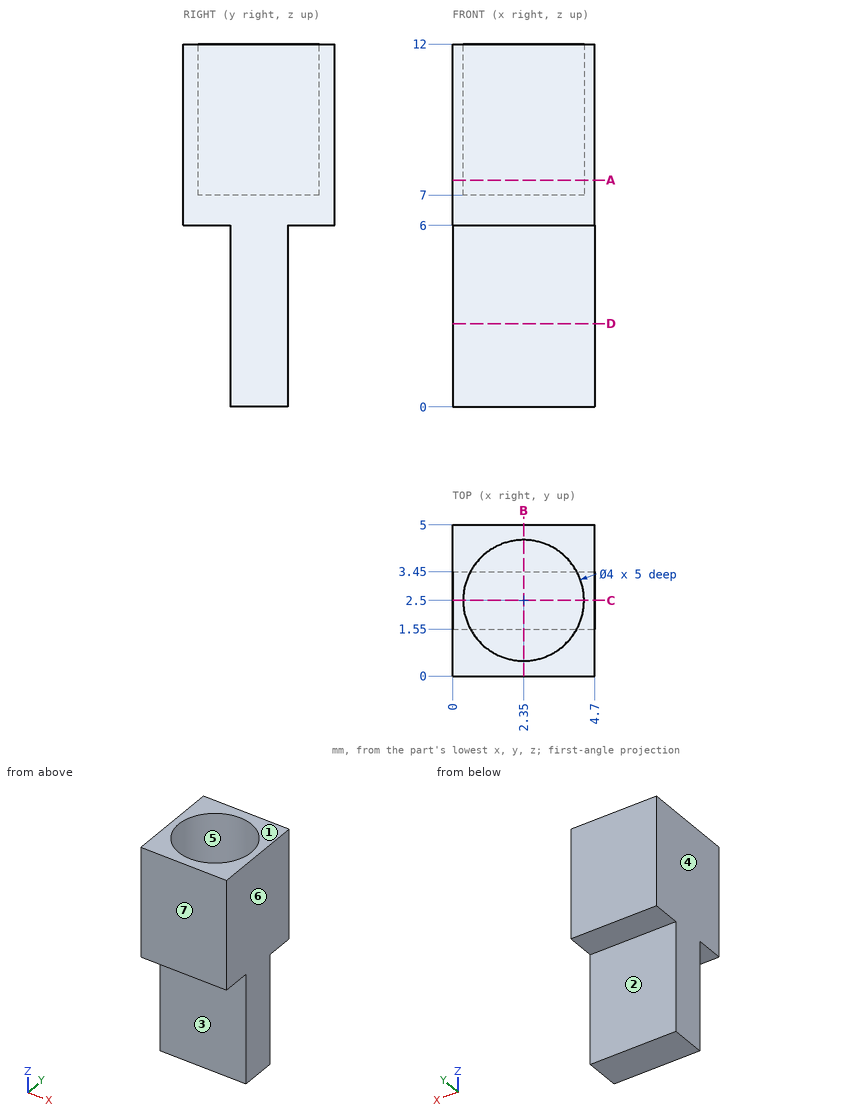
Here's the drawing with two shaded views (mm, measured from the low corner). I have some questions. A direction names the side the tool comes from. Give positions to 0.01 mm unless a question says otherwise; leave off trailing zeros. Order: outer loops, then holes, each group sorted by start corner. A loop starts at its lowest first (then second) coordinate and runs counter-clockwise, first axis right, second up. Notation, with made-up numbers: (-14.75, 83.25) -> (7.25, 83.25) arc R24 cw to (7.25, 98.25) -> close; hole circle Ø8 at (16.25, -6). An arc over 180 degrees is marked (long way). One line per item, written item: value. Start each with the question number.
1. Imagine slicing it at D-D, the plane z = 2.75. List the corners of the cut face in (x, y) for me.
2. Imagine slicing it at A-A, the plane z = 7.5. List the corners of the cut face in (x, y) for me.
3. I need wall thicknesses on probe 1 along Y at (x, z) = (2.35, 11); probe 2 along Z at (x, y) = (2.8, 0.7); probe 3 along Y at (x, z) = (0.8, 3.5). Which ranges of each line are inside material? Lowest first, please. Write a range as from..to.
4. For the marked faces 1, 2 and 3, which set-ups out of +Z, -Z, +X, -X, +Y, -Y let a thin tool reach every point of the face, with its end or its side?
5. Will these pins go through, and if not, where does the flat tip stop? pin 1 Ø1.5 at (x, y) = (3.5, 4.5) entering from -Z; pin 2 Ø2 at (x, z) = (3.5, 2.5) entering from +Y.
6. We'd pull the mould along X, two halves only. Please class the marked faces 4, 5, 6 and 7: released by +X, released by -X, zero draft, split by the parting line, or undercut.
7. Imagine slicing it at B-B, the plane x = 2.35. List the corners of the cut face in (y, z) for me.
8. Imagine slicing it at C-C, the plane y = 2.5. List the corners of the cut face in (x, z) for me.
Values follow:
1. outline: (0, 1.55) -> (4.7, 1.55) -> (4.7, 3.45) -> (0, 3.45) -> close
2. outline: (0, 0) -> (4.7, 0) -> (4.7, 5) -> (0, 5) -> close; hole circle Ø4 at (2.35, 2.5)
3. probe 1: y = 0..0.5, 4.5..5
3. probe 2: z = 6..7
3. probe 3: y = 1.55..3.45
4. face 1: +Z, +X, -X, +Y, -Y
4. face 2: -Z, +X, -X, +Y
4. face 3: -Z, +X, -X, -Y
5. pin 1: stops at z = 6
5. pin 2: stops at y = 3.45
6. face 4: released by -X
6. face 5: undercut
6. face 6: released by +X
6. face 7: zero draft
7. outline: (0, 6) -> (1.55, 6) -> (1.55, 0) -> (3.45, 0) -> (3.45, 6) -> (5, 6) -> (5, 12) -> (4.5, 12) -> (4.5, 7) -> (0.5, 7) -> (0.5, 12) -> (0, 12) -> close
8. outline: (0, 0) -> (4.7, 0) -> (4.7, 12) -> (4.35, 12) -> (4.35, 7) -> (0.35, 7) -> (0.35, 12) -> (0, 12) -> close
